Autodesk Inventor part; units mm, degrees
ref_plane "Work Plane1" through (-1.5, 1, -12.5) normal (-1, 0, 0) x (0, 0, 1)
ref_plane "YZ Plane" through (0, 0, 0) normal (1, 0, 0) x (0, 1, 0)
ref_plane "XZ Plane" through (0, 0, 0) normal (0, 1, 0) x (-1, 0, 0)
sketch "Sketch1" plane through (0, 0, 0) normal (0, 0, 1) x (1, 0, 0)
  line L0 (-6, 1) -> (6, 1)
  line L1 (6, 1) -> (6, -1)
  line L2 (6, -1) -> (-6, -1)
  line L3 (-6, -1) -> (-6, 1)
  line L4 (-6, 1) -> (6, -1) construction
  line L5 (6, 1) -> (-6, -1) construction
  line L6 (-6, -1) -> (-6, -3)
  line L7 (6, -1) -> (6, -3)
  arc A0 (6, -3) -> (-6, -3) centre (0, -11) ccw
  point P0 (0, 0)
  dimension "d0" = 12
  dimension "d1" = 2
  dimension "d2" = 2
  dimension "d3" = 2
extrude "Extrusion1" add sketch "Sketch1" against normal blind 25
sketch "Sketch2" plane through (-6, 1, 0) normal (0, 1, 0) x (1, 0, 0)
  line L0 (12, 0) -> (12, 25)
  line L1 (0, 0) -> (0, 25)
  line L2 (0, 0) -> (0, 2.5)
  line L3 (12, 0) -> (12, 2.5)
  line L4 (0, 25) -> (0, 22.5)
  line L5 (12, 25) -> (12, 22.5)
  line L6 (0, 2.5) -> (4.5, 2.5)
  line L7 (4.5, 2.5) -> (4.5, 22.5)
  line L8 (4.5, 22.5) -> (0, 22.5)
  line L9 (0, 22.5) -> (0, 2.5)
  line L10 (12, 2.5) -> (7.5, 2.5)
  line L11 (7.5, 2.5) -> (7.5, 22.5)
  line L12 (7.5, 22.5) -> (12, 22.5)
  line L13 (12, 22.5) -> (12, 2.5)
  point P0 (6, 0)
  dimension "d6" = 2.5
  dimension "d7" = 2.5
  dimension "d8" = 2.5
  dimension "d9" = 2.5
  dimension "d10" = 12
  dimension "d11" = 4.5
  dimension "d12" = 4.5
extrude "Extrusion2" cut sketch "Sketch2" against normal blind 25
sketch "Sketch3" plane through (-6, 1, 0) normal (0, 1, 0) x (1, 0, 0)
  line L0 (7.5, 2.5) -> (7.5, 22.5)
  line L1 (4.5, 22.5) -> (4.5, 2.5)
  line L2 (0, 0) -> (0, 2.5)
  line L3 (4.5, 2.5) -> (4.5, 3.5)
  line L4 (7.5, 2.5) -> (7.5, 3.5)
  line L5 (4.5, 3.5) -> (4.5, 5)
  line L6 (4.5, 5) -> (5, 5)
  line L7 (5, 5) -> (5, 3.5)
  line L8 (5, 3.5) -> (4.5, 3.5)
  line L9 (7.5, 3.5) -> (7.5, 5)
  line L10 (7.5, 5) -> (7, 5)
  line L11 (7, 5) -> (7, 3.5)
  line L12 (7, 3.5) -> (7.5, 3.5)
  line L13 (4.5, 2.5) -> (4.5, 7)
  line L14 (4.5, 7) -> (0, 7)
  line L15 (0, 7) -> (0, 8.5)
  line L16 (0, 8.5) -> (4.5, 8.5)
  line L17 (7.5, 7) -> (12, 7)
  line L18 (12, 7) -> (12, 8.5)
  line L19 (12, 8.5) -> (7.5, 8.5)
  line L20 (4.5, 7) -> (4.5, 21)
  line L21 (7.5, 7) -> (7.5, 21)
  line L22 (4.5, 21) -> (7.5, 21)
  line L23 (7.5, 21) -> (7.5, 22.5)
  line L24 (7.5, 22.5) -> (4.5, 22.5)
  line L25 (4.5, 22.5) -> (4.5, 21)
  line L26 (4.5, 21) -> (3.5, 21)
  line L27 (3.5, 21) -> (3.5, 11)
  line L28 (3.5, 11) -> (4.5, 11)
  line L29 (4.5, 11) -> (4.5, 21)
  line L30 (7.5, 21) -> (8.5, 21)
  line L31 (8.5, 21) -> (8.5, 11)
  line L32 (8.5, 11) -> (7.5, 11)
  line L33 (7.5, 11) -> (7.5, 21)
  line L34 (3.5, 21) -> (4.5, 22.5)
  line L35 (7.5, 22.5) -> (8.5, 21)
  line L36 (7.5, 5) -> (8, 5)
  line L37 (8, 5) -> (8, 3.5)
  line L38 (8, 3.5) -> (7.5, 3.5)
  line L39 (4.5, 5) -> (4, 5)
  line L40 (4, 5) -> (4, 3.5)
  line L41 (4, 3.5) -> (5, 3.5)
  point P0 (12, 25)
  point P1 (12, 0)
  point P2 (6, 0)
  dimension "d15" = 1
  dimension "d16" = 1.5
  dimension "d17" = 0.5
  dimension "d18" = 0.5
  dimension "d19" = 4.5
  dimension "d20" = 1.5
  dimension "d21" = 14
  dimension "d22" = 4.5
  dimension "d23" = 4.5
  dimension "d24" = 14
  dimension "d25" = 25
  dimension "d26" = 1.5
  dimension "d29" = 1
  dimension "d30" = 10
  dimension "d31" = 1
  dimension "d34" = 0.5
  dimension "d35" = 0.5
  dimension "d50" = 10
extrude "Extrusion3" add sketch "Sketch3" along normal blind 4 contours L0 L30 L31 L32 | L22 L1 L24 L0 | L0 L35 L30 | L26 L34 L1 | L1 L28 L27 L26
ref_plane "Work Plane1" through (-1.5, 1, -12.5) normal (-1, 0, 0) x (0, 0, 1)
sketch "Sketch8" plane through (-2.5, -1.3175, -11) normal (-1, 0, 0) x (0, 0, 1)
  line L0 (-10, 0) -> (0, 6.3175)
  line L1 (-10, 6.3175) -> (-11.5, 6.3175)
  line L2 (0, 0) -> (-10, 0)
  line L3 (-10, 6.3175) -> (0, 0)
  line L4 (-4, 1.1588) -> (-4, 5.1588)
  line L5 (-6, 1.1588) -> (-4, 5.1588) construction
  line L6 (-4, 1.1588) -> (-6, 5.1588) construction
  line L7 (-5, 3.1588) -> (-2, 3.1588)
  line L8 (-3, 5.1588) -> (-1, 5.1588)
  line L9 (-1, 5.1588) -> (-1, 1.1588)
  line L10 (-1, 1.1588) -> (-3, 1.1588)
  line L11 (-3, 1.1588) -> (-3, 5.1588)
  line L12 (-3, 5.1588) -> (-1, 1.1588) construction
  line L13 (-1, 5.1588) -> (-3, 1.1588) construction
  line L14 (0, 2.3175) -> (0, 6.3175)
  line L15 (-10, 6.3175) -> (0, 6.3175)
  line L16 (-6, 5.1588) -> (-3, 5.1588)
  point P0 (11, 1.3175)
  dimension "d51" = 2
  dimension "d52" = 4
  dimension "d103" = 3
  dimension "d104" = 2
  dimension "d105" = 4
extrude "Extrusion8" add sketch "Sketch8" along normal blind 3 contours L10 L11 L3 | L3 L11 L0 L8 L9 L10 | L11 L8 L0
sketch "Sketch9" plane through (2.5, -1.3175, -21) normal (1, 0, 0) x (0, 0, -1)
  line L0 (-10, 6.3175) -> (0, 0)
  line L1 (0, 2.3175) -> (0, 6.3175)
  line L2 (0, 0) -> (-10, 0)
  line L3 (0, 6.3175) -> (-10, 0)
  line L4 (-6, 5.1588) -> (-6, 1.1588)
  line L5 (-4, 5.1588) -> (-6, 1.1588) construction
  line L6 (-6, 5.1588) -> (-4, 1.1588) construction
  line L7 (-5, 3.1588) -> (-8, 3.1588)
  line L8 (-9, 2.3175) -> (-9, 1.1588)
  line L9 (-7, 5.1588) -> (-9, 5.1588)
  line L10 (-9, 5.1588) -> (-9, 1.1588)
  line L11 (-9, 1.1588) -> (-7, 1.1588)
  line L12 (-7, 1.1588) -> (-7, 5.1588)
  line L13 (-7, 5.1588) -> (-9, 1.1588) construction
  line L14 (-9, 5.1588) -> (-7, 1.1588) construction
  point P0 (-21, 1.3175)
  dimension "d55" = 2
  dimension "d56" = 4
  dimension "d106" = 3
extrude "Extrusion9" add sketch "Sketch9" along normal blind 3 contours L12 L3 L11 L8 L10 L9 L0 | L0 L9 L12 | L12 L11 L3
ref_plane "Work Plane2" through (-2, 1, -11) normal (1, 0, 0) x (0, 0, -1)
sketch "Sketch12" plane through (-2, 1, -11) normal (1, 0, 0) x (0, 0, -1)
  line L0 (11.5, 0) -> (11.5, 4)
  line L1 (14, -4) -> (14, 0)
  line L2 (14, 0) -> (11.5, 4)
  line L3 (11.5, 0) -> (14, 0)
  line L4 (14, 0) -> (11.5, 0)
  line L5 (11.5, 4) -> (12.8115, 3.0819) construction
  line L6 (12.8115, 3.0819) -> (14.0937, 1.3588) construction
  line L7 (14.0937, 1.3588) -> (14, 0) construction
  spline S0 degree 3 poles (11.5, 4) (12.8115, 3.0819) (14.0937, 1.3588) (14, 0) knots 1 1 1 1 2 2 2 2
  point P0 (-11, -1)
extrude "Extrusion12" add sketch "Sketch12" along normal up to surface (3.5 mm away)
sketch "Sketch15" plane through (2.5, -1.3175, -21) normal (1, 0, 0) x (0, 0, -1)
  line L0 (1.5, 2.3175) -> (4, 2.3175)
  line L1 (1.5, 2.3175) -> (1.5, 6.3175)
  line L2 (4, 2.3175) -> (1.5, 2.3175)
  line L3 (1.5, 2.3175) -> (1.5, 3.3175)
  circle A0 centre (1.5, 3.3175) radius 1.3
  point P0 (-21, 1.3175)
  dimension "d77" = 1
  dimension "d78" = 2.6
extrude "Extrusion14" cut sketch "Sketch15" against normal up to surface (12 mm away) from surface at 3.5
sketch "Sketch16" plane through (-6, 5, 0) normal (0, 1, 0) x (1, 0, 0)
  line L0 (3.5, 11) -> (4.5, 11)
  line L1 (4.5, 11) -> (4.5, 21)
  line L2 (7.5, 21) -> (7.5, 11)
  line L3 (7.5, 11) -> (8.5, 11)
  line L4 (4.5, 11) -> (4.3, 11)
  line L5 (4.3, 11) -> (4.3, 21)
  line L6 (4.3, 21) -> (4.5, 21)
  line L7 (7.5, 11) -> (7.5, 21)
  line L8 (7.5, 11) -> (7.7, 11)
  line L9 (7.7, 11) -> (7.7, 21)
  line L10 (7.7, 21) -> (7.5, 21)
  line L11 (7.5, 21) -> (7.5, 11)
  point P0 (6, 0)
  dimension "d81" = 0.2
  dimension "d82" = 0.2
  dimension "d83" = 0.2
extrude "Extrusion15" cut sketch "Sketch16" against normal up to surface (4 mm away)
sketch "Sketch17" plane through (1.5, -1.1131, -2.5) normal (1, 0, 0) x (0, 0, -1)
  line L0 (0, 2.1131) -> (18.5, 2.1131)
  line L1 (-2.5, 2.1131) -> (0, 2.1131)
  line L2 (-2.5, 2.1131) -> (-2.5, 3.1131)
  line L3 (-2.5, 3.1131) -> (-1.5, 3.1131)
  line L4 (-1.5, 3.1131) -> (1, 3.1131)
  line L5 (1, 3.1131) -> (2, 3.1131)
  line L6 (-0.25, 3.1131) -> (-0.25, 4.3631)
  line L7 (-0.25, 4.3631) -> (-0.25, 5.3631)
  line L8 (-2.5, 2.1131) -> (2, 2.1131)
  line L9 (2, 3.1131) -> (2, 2.1131)
  arc A0 (2, 3.1131) -> (-2.5, 3.1131) centre (-0.25, 3.1131) ccw
  dimension "d94" = 1
  dimension "d95" = 1
  dimension "d96" = 2.5
  dimension "d97" = 1
  dimension "d98" = 1.25
  dimension "d99" = 1
extrude "Extrusion16" add sketch "Sketch17" against normal up to surface (3 mm away)
sketch "Sketch19" plane through (6, -3, 0) normal (1, 0, 0) x (0, 0, -1)
  arc A0 (4.5, 5) -> (0, 5) centre (2.25, 5) ccw
  circle A1 centre (2.25, 5) radius 1.25
  point P0 (0, 3)
  dimension "d100" = 2.5
extrude "Extrusion17" cut sketch "Sketch19" against normal up to surface (12 mm away)
equation "\"d7\" = d6"
equation "\"d8\" = d6"
equation "\"d9\" = d6"
equation "\"d12\" = d11"
equation "\"d18\" = d17"
equation "\"d22\" = d23"
equation "\"d24\" = d21"
equation "\"d31\" = d29"
equation "\"d50\" = d30"
equation "\"d82\" = d81"
properties part number "back_pack_3.1"
Input: part model. Units: mm. Frame: model coordinates. A direction names the side the tool comes from. Coordinates: 2 decimals unless noted, no trailing zeros. Loops run counter-clockwise (first coordinate to the right, second up) from the corner with the lowest first, then second, coordinate; pieces in that order, holes last.
(1) Material intervals for probe 1 along X at (y, z) = (4.75, -16.25); probe 2 along Z at (x, y) = (-4, -1.75); probe 3 along Z at (x, y) = (1.25, 2), sorted ascending.
(2) Section B-B on x = -5. Return the cut outline in (y, z).
(3) Pull-direction query (Y, two-part tool) for faces 4 (the face through (1.5, 3, -24)), 5 (the face through (0.08, 0.78, -1.98)), 6 (the face through (4, 1, -24)); classes: released by +Y, released by -Y, zero draft, split by the parting line, or undercut.
(4) Set-up query: faces 1 (the face through (2.5, 0, -13)), 2 (the face through (0, 1, -13)), 3 (the face through (-4, 1, -1)). Return all of +Z, -Z, +X, -X, +Y, -Y with unobstructed straight access to the full face (end or side cutting, diameter ignored); none if empty.
(5) Section C-C on x = 1. Count the separate pieces of the cut face and the enclosed holes in it, then the cut area to 3 significant figures.
(6) First-contact query: pin 1 Ø0.9 at (x, y) = (-2, 2.5) entering from +Z; pin 2 Ø1.6 at (x, z) = (-4.5, -12.5) entering from -Y; pin 3 Ø3 at (x, z) = (-3.5, -19.5) entering from -Y. Flat tips, straight axial feed; report the tip coordinate or a pass-through.
(7) Section A-A on z = -2.25. Return the cut outline in (x, y), then the cut area to 3 significant figures.
Data:
1. probe 1: x = -2.5 to -1.7, 1.7 to 2.5
1. probe 2: z = -25 to -22.5, -2.5 to 0
1. probe 3: z = -24.86 to -23.8, -21.2 to -21, -4.5 to -3.5, -1 to 0
2. outline: (-2.34, -25) - (1, -25) - (1, -23.33) arc R1.3 cw to (0.7, -22.5) - (-2.34, -22.5) - close; (-2.34, -2.5) - (0.78, -2.5) arc R1.25 cw to (1, -1.5) - (1, 0) - (-2.34, 0) - close; (-0.16, -14) - (3.84, -14) - (3.84, -12) - (-0.16, -12) - close
3. face 4: zero draft
3. face 5: undercut
3. face 6: released by +Y
4. face 1: -Y
4. face 2: +Y
4. face 3: +Z, -X, +Y
5. separate pieces: 1
5. enclosed holes: 2
5. area: 66.2 mm2
6. pin 1: stops at z = -11
6. pin 2: stops at y = -0.16
6. pin 3: stops at y = 1
7. outline: (-6, -3) arc R10 cw to (6, -3) - (6, 0.75) - (-6, 0.75) - close; (-1.5, 3.25) - (1.5, 3.25) - (1.5, 4.25) - (-1.5, 4.25) - close
7. area: 31.6 mm2
